The figure shows three views and two pictorial views of one solid part (mm, origin at its lowest corner). Answer the questions. Coordinates: 2 decimals unless noted, no trailing zeros. Order: outer loops, then holes, each group sorted by start corner. A loop starts at its lowest first (then second) coordinate and runs counter-clockwise, first axis right, second up. Notation, with made-up numbers: (-4.5, 10.5) -> (37.5, 10.5) arc R16 ccw to (37.5, 27.5) -> close; hole circle Ø1 at (84.25, 28.5). An arc over 180 degrees is marked (long way). Return JSON: item names as keys, results as strings.
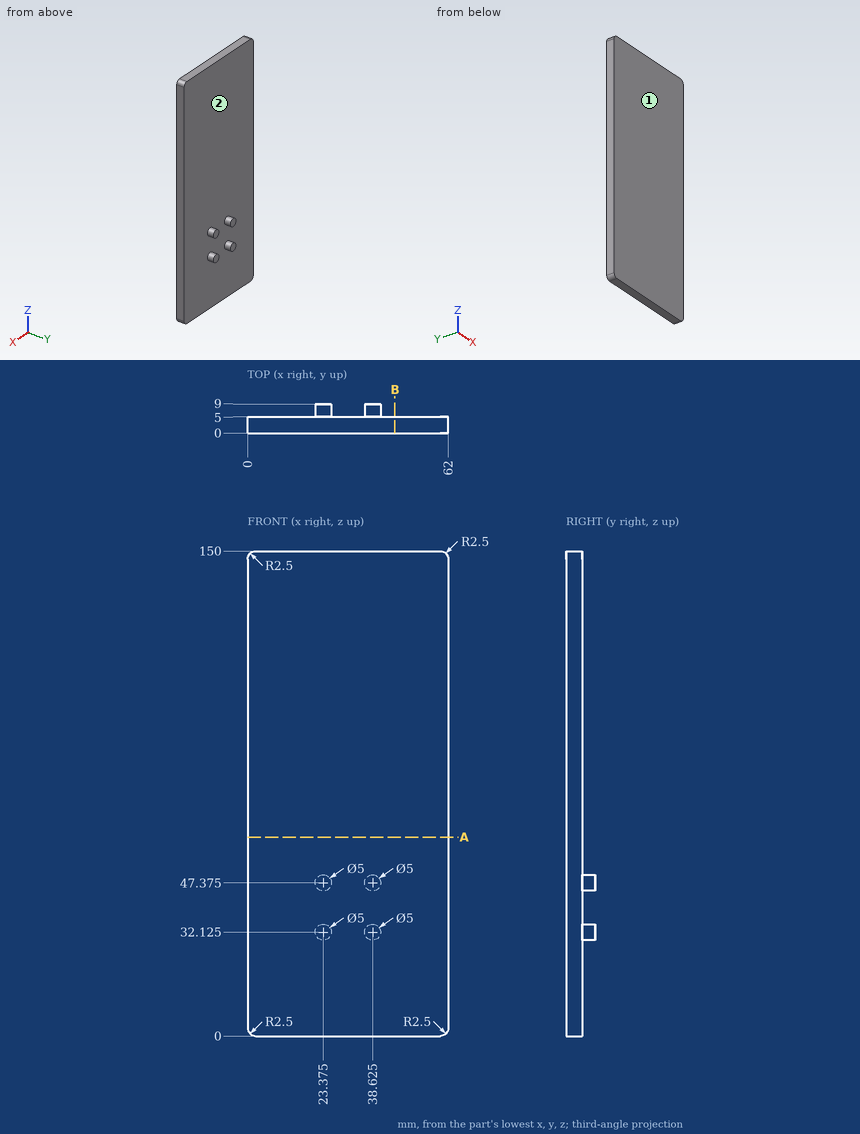
Item 1: The part is cut by section B-B on x = 45.5. Determine the outline of the cut face in (y, z).
Answer list:
{"outline": "(0, 0) -> (5, 0) -> (5, 150) -> (0, 150) -> close"}
Item 2: Find the intervals of material crossed by probe 1 along Y at (x, z) = (22.5, 44), in increasing order.
Answer list:
{"probe 1": "0 to 5"}
Item 3: Determine the mould class of the marked faces 1 and 2 for opening direction Y: pulls with the +Y half, pulls with the -Y half, needs draft (parallel to the pull), parting line crosses it, or undercut.
Answer list:
{"face 1": "pulls with the -Y half", "face 2": "pulls with the +Y half"}
Item 4: The part is cut by section A-A on z = 61.5. Determine the outline of the cut face in (x, y), plus the area to 3 significant figures.
Answer list:
{"outline": "(0, 0) -> (62, 0) -> (62, 5) -> (0, 5) -> close", "area": "310 mm2"}
